The listing builds one solid part. Answer for the finished solid, in the listing's coordinates (mm). A direction names the side the tool comes from. Coordinates: 2 decimals unless noted, no trailing zeros. Loops run counter-clockwise (first coordinate to the right, second up) from the corner with the lowest first, then second, coordinate; pieces in that order, holes last. Notation, with made-up numbers: (-33, -7.5) - (-15, -7.5) arc R18 ccw to (-15, 12.5) - close; hole circle Ø7 at (29.5, 39.5). An arc over 180 degrees is marked (long way). Put each result on its own line as item: value.
```python
from build123d import *
from build123d.topology import SkipClean

# Parameters (mm, degrees)
SKETCH_1_W                       = 300
SKETCH_1_H                       = 135
SKETCH_1_R                       = 3
SM_BASE_FLANGE_1_DEPTH           = 0.7
SM_EDGE_FLANGE_1_STRIP_W         = 3.2
SM_EDGE_FLANGE_1_STRIP_H         = 0.7
SM_EDGE_FLANGE_1_STRIP_CUT_DEPTH = 300
SM_EDGE_FLANGE_1_DEPTH           = 300
SM_EDGE_FLANGE_2_STRIP_W         = 3.2
SM_EDGE_FLANGE_2_STRIP_H         = 0.7
SM_EDGE_FLANGE_2_STRIP_CUT_DEPTH = 300
SM_EDGE_FLANGE_2_DEPTH           = 300
MOVE_START                       = -0.5
MOVE_BODY_1_OUTLINE_W            = 300
MOVE_BODY_1_OUTLINE_H            = 134.3
MOVE_BODY_1_OUTLINE_R            = 3
MOVE_BODY_1_DEPTH                = 0.5
MOVE_START_2                     = -6
MOVE_BODY_1_2_OUTLINE_W          = 300
MOVE_BODY_1_2_OUTLINE_H          = 6
MOVE_BODY_1_2_DEPTH              = 4.6
MOVE_START_3                     = -1.343604
MOVE_BODY_1_3_OUTLINE_W          = 300
MOVE_BODY_1_3_OUTLINE_H          = 134.3
MOVE_BODY_1_3_OUTLINE_R          = 3
MOVE_BODY_1_3_DEPTH              = 0.643604
MOVE_BODY_1_4_OUTLINE_W          = 300
MOVE_BODY_1_4_OUTLINE_H          = 0.7
MOVE_BODY_1_4_DEPTH              = 4.2
MOVE_START_4                     = -1.4
MOVE_BODY_1_5_OUTLINE_W          = 300
MOVE_BODY_1_5_OUTLINE_H          = 134.3
MOVE_BODY_1_5_OUTLINE_R          = 3
MOVE_BODY_1_5_DEPTH              = 0.056396
MOVE_START_5                     = 3.7
MOVE_BODY_1_6_OUTLINE_W          = 300
MOVE_BODY_1_6_OUTLINE_H          = 6
MOVE_BODY_1_6_DEPTH              = 0.9
MOVE_START_6                     = -0.7
MOVE_BODY_1_7_OUTLINE_W          = 300
MOVE_BODY_1_7_OUTLINE_H          = 0.7
MOVE_BODY_1_7_DEPTH              = 0.2
MOVE_START_7                     = -151
MOVE_BODY_1_8_DEPTH              = 301


with BuildPart() as part:
    # 基体-法兰1: sheet metal written as solids
    # 草图1 → 基体-法兰1 (new body)
    with BuildSketch(Plane(origin=(0, 0, 0), x_dir=(1, 0, 0), z_dir=(0, 1, 0))):
        Rectangle(SKETCH_1_W, SKETCH_1_H)
        with Locations(Location((-144.5, -59.5, 0), (0, 0, 270))):
            Circle(SKETCH_1_R, mode=Mode.SUBTRACT)
        with Locations(Location((-144.5, -9.5, 0), (0, 0, 270))):
            Circle(SKETCH_1_R, mode=Mode.SUBTRACT)
        with Locations(Location((-144.5, 0.5, 0), (0, 0, 270))):
            Circle(SKETCH_1_R, mode=Mode.SUBTRACT)
        with Locations(Location((-144.5, 50.5, 0), (0, 0, 270))):
            Circle(SKETCH_1_R, mode=Mode.SUBTRACT)
        with Locations(Location((0, -9.5, 0), (0, 0, 270))):
            Circle(SKETCH_1_R, mode=Mode.SUBTRACT)
        with Locations(Location((0, 0.5, 0), (0, 0, 270))):
            Circle(SKETCH_1_R, mode=Mode.SUBTRACT)
        with Locations(Location((144.5, -59.5, 0), (0, 0, 90))):
            Circle(SKETCH_1_R, mode=Mode.SUBTRACT)
        with Locations(Location((144.5, -9.5, 0), (0, 0, 90))):
            Circle(SKETCH_1_R, mode=Mode.SUBTRACT)
        with Locations(Location((144.5, 0.5, 0), (0, 0, 90))):
            Circle(SKETCH_1_R, mode=Mode.SUBTRACT)
        with Locations(Location((144.5, 50.5, 0), (0, 0, 90))):
            Circle(SKETCH_1_R, mode=Mode.SUBTRACT)
    extrude(amount=-SM_BASE_FLANGE_1_DEPTH)

    # 边线-法兰1: sheet metal written as solids
    # 边线-法兰1 strip (on a plane across the edge) → 边线-法兰1 strip cut (cut)
    with BuildSketch(Plane(origin=(-150, -0.7, -67.5), x_dir=(0, 0, 1), z_dir=(1, 0, 0))):
        with Locations((-0.7, -0.35)):
            Rectangle(SM_EDGE_FLANGE_1_STRIP_W, SM_EDGE_FLANGE_1_STRIP_H)
    extrude(amount=SM_EDGE_FLANGE_1_STRIP_CUT_DEPTH, mode=Mode.SUBTRACT)

    # 边线-法兰1 section (on a plane across the edge) → 边线-法兰1 (add)
    with BuildSketch(Plane(origin=(-150, -0.7, -67.5), x_dir=(0, 0, 1), z_dir=(1, 0, 0))):
        with BuildLine():
            Line((0, 0.2), (0, 5.3))
            Line((0, 5.3), (0.7, 5.3))
            Line((0.7, 5.3), (0.7, 0.2))
            ThreePointArc((0.7, 0.2), (0.758578644, 0.058578644), (0.9, 0))
            Line((0.9, 0), (0.9, -0.7))
            ThreePointArc((0.9, -0.7), (0.263603897, -0.436396103), (0, 0.2))
        make_face()
    extrude(amount=SM_EDGE_FLANGE_1_DEPTH)

    # 边线-法兰2: sheet metal written as solids
    # 边线-法兰2 strip (on a plane across the edge) → 边线-法兰2 strip cut (cut)
    with BuildSketch(Plane(origin=(150, -6, -67.5), x_dir=(0, 1, 0), z_dir=(-1, 0, 0))):
        with Locations((-0.7, -0.35)):
            Rectangle(SM_EDGE_FLANGE_2_STRIP_W, SM_EDGE_FLANGE_2_STRIP_H)
    extrude(amount=SM_EDGE_FLANGE_2_STRIP_CUT_DEPTH, mode=Mode.SUBTRACT)

    # 边线-法兰2 section (on a plane across the edge) → 边线-法兰2 (add)
    with BuildSketch(Plane(origin=(150, -6, -67.5), x_dir=(0, 1, 0), z_dir=(-1, 0, 0))):
        with BuildLine():
            Line((0, 0.2), (0, 5.3))
            Line((0, 5.3), (0.7, 5.3))
            Line((0.7, 5.3), (0.7, 0.2))
            ThreePointArc((0.7, 0.2), (0.758578644, 0.058578644), (0.9, 0))
            Line((0.9, 0), (0.9, -0.7))
            ThreePointArc((0.9, -0.7), (0.263603897, -0.436396103), (0, 0.2))
        make_face()
    extrude(amount=SM_EDGE_FLANGE_2_DEPTH)

    # Move Body 1: read off the stored shape, not the designer's step
    # Move Body 1 outline → Move Body 1 (cut)
    with BuildSketch(Plane(origin=(0, 0, 0), x_dir=(1, 0, 0), z_dir=(0, 1, 0)).offset(MOVE_START)):
        with Locations((0, -0.35)):
            Rectangle(MOVE_BODY_1_OUTLINE_W, MOVE_BODY_1_OUTLINE_H)
        with Locations((-144.5, -59.5)):
            Circle(MOVE_BODY_1_OUTLINE_R, mode=Mode.SUBTRACT)
        with Locations((-144.5, -9.5)):
            Circle(MOVE_BODY_1_OUTLINE_R, mode=Mode.SUBTRACT)
        with Locations((-144.5, 0.5)):
            Circle(MOVE_BODY_1_OUTLINE_R, mode=Mode.SUBTRACT)
        with Locations((144.5, -59.5)):
            Circle(MOVE_BODY_1_OUTLINE_R, mode=Mode.SUBTRACT)
        with Locations((0, -9.5)):
            Circle(MOVE_BODY_1_OUTLINE_R, mode=Mode.SUBTRACT)
        with Locations((0, 0.5)):
            Circle(MOVE_BODY_1_OUTLINE_R, mode=Mode.SUBTRACT)
        with Locations((144.5, -9.5)):
            Circle(MOVE_BODY_1_OUTLINE_R, mode=Mode.SUBTRACT)
        with Locations((144.5, 0.5)):
            Circle(MOVE_BODY_1_OUTLINE_R, mode=Mode.SUBTRACT)
        with Locations((-144.5, 50.5)):
            Circle(MOVE_BODY_1_OUTLINE_R, mode=Mode.SUBTRACT)
        with Locations((144.5, 50.5)):
            Circle(MOVE_BODY_1_OUTLINE_R, mode=Mode.SUBTRACT)
    extrude(amount=MOVE_BODY_1_DEPTH, mode=Mode.SUBTRACT)

    # Move Body 1 2 outline → Move Body 1 2 (cut)
    with BuildSketch(Plane(origin=(0, 0, 0), x_dir=(1, 0, 0), z_dir=(0, 1, 0)).offset(MOVE_START_2)):
        with Locations((0, 69.8)):
            Rectangle(MOVE_BODY_1_2_OUTLINE_W, MOVE_BODY_1_2_OUTLINE_H)
    extrude(amount=MOVE_BODY_1_2_DEPTH, mode=Mode.SUBTRACT)

    # Move Body 1 3 outline → Move Body 1 3 (add)
    with SkipClean():  # the faces are left unmerged after this step: merging them gives an invalid solid
        with BuildSketch(Plane(origin=(0, 0, 0), x_dir=(1, 0, 0), z_dir=(0, 1, 0)).offset(MOVE_START_3)):
            with Locations((0, -0.35)):
                Rectangle(MOVE_BODY_1_3_OUTLINE_W, MOVE_BODY_1_3_OUTLINE_H)
            with Locations((-144.5, -59.5)):
                Circle(MOVE_BODY_1_3_OUTLINE_R, mode=Mode.SUBTRACT)
            with Locations((-144.5, -9.5)):
                Circle(MOVE_BODY_1_3_OUTLINE_R, mode=Mode.SUBTRACT)
            with Locations((-144.5, 0.5)):
                Circle(MOVE_BODY_1_3_OUTLINE_R, mode=Mode.SUBTRACT)
            with Locations((144.5, -59.5)):
                Circle(MOVE_BODY_1_3_OUTLINE_R, mode=Mode.SUBTRACT)
            with Locations((0, -9.5)):
                Circle(MOVE_BODY_1_3_OUTLINE_R, mode=Mode.SUBTRACT)
            with Locations((0, 0.5)):
                Circle(MOVE_BODY_1_3_OUTLINE_R, mode=Mode.SUBTRACT)
            with Locations((144.5, -9.5)):
                Circle(MOVE_BODY_1_3_OUTLINE_R, mode=Mode.SUBTRACT)
            with Locations((144.5, 0.5)):
                Circle(MOVE_BODY_1_3_OUTLINE_R, mode=Mode.SUBTRACT)
            with Locations((-144.5, 50.5)):
                Circle(MOVE_BODY_1_3_OUTLINE_R, mode=Mode.SUBTRACT)
            with Locations((144.5, 50.5)):
                Circle(MOVE_BODY_1_3_OUTLINE_R, mode=Mode.SUBTRACT)
        extrude(amount=MOVE_BODY_1_3_DEPTH)

    # Move Body 1 4 outline → Move Body 1 4 (add)
    with SkipClean():  # the faces are left unmerged after this step: merging them gives an invalid solid
        with BuildSketch(Plane(origin=(0, 0, 0), x_dir=(1, 0, 0), z_dir=(0, 1, 0)).offset(MOVE_START)):
            with Locations((0, 67.15)):
                Rectangle(MOVE_BODY_1_4_OUTLINE_W, MOVE_BODY_1_4_OUTLINE_H)
        extrude(amount=MOVE_BODY_1_4_DEPTH)

    # Move Body 1 5 outline → Move Body 1 5 (add)
    with SkipClean():  # the faces are left unmerged after this step: merging them gives an invalid solid
        with BuildSketch(Plane(origin=(0, 0, 0), x_dir=(1, 0, 0), z_dir=(0, 1, 0)).offset(MOVE_START_4)):
            with Locations((0, -0.35)):
                Rectangle(MOVE_BODY_1_5_OUTLINE_W, MOVE_BODY_1_5_OUTLINE_H)
            with Locations((-144.5, -59.5)):
                Circle(MOVE_BODY_1_5_OUTLINE_R, mode=Mode.SUBTRACT)
            with Locations((-144.5, -9.5)):
                Circle(MOVE_BODY_1_5_OUTLINE_R, mode=Mode.SUBTRACT)
            with Locations((-144.5, 0.5)):
                Circle(MOVE_BODY_1_5_OUTLINE_R, mode=Mode.SUBTRACT)
            with Locations((144.5, -59.5)):
                Circle(MOVE_BODY_1_5_OUTLINE_R, mode=Mode.SUBTRACT)
            with Locations((0, -9.5)):
                Circle(MOVE_BODY_1_5_OUTLINE_R, mode=Mode.SUBTRACT)
            with Locations((0, 0.5)):
                Circle(MOVE_BODY_1_5_OUTLINE_R, mode=Mode.SUBTRACT)
            with Locations((144.5, -9.5)):
                Circle(MOVE_BODY_1_5_OUTLINE_R, mode=Mode.SUBTRACT)
            with Locations((144.5, 0.5)):
                Circle(MOVE_BODY_1_5_OUTLINE_R, mode=Mode.SUBTRACT)
            with Locations((-144.5, 50.5)):
                Circle(MOVE_BODY_1_5_OUTLINE_R, mode=Mode.SUBTRACT)
            with Locations((144.5, 50.5)):
                Circle(MOVE_BODY_1_5_OUTLINE_R, mode=Mode.SUBTRACT)
        extrude(amount=MOVE_BODY_1_5_DEPTH)

    # Move Body 1 6 outline → Move Body 1 6 (add)
    with SkipClean():  # the faces are left unmerged after this step: merging them gives an invalid solid
        with BuildSketch(Plane(origin=(0, 0, 0), x_dir=(1, 0, 0), z_dir=(0, 1, 0)).offset(MOVE_START_5)):
            with Locations((0, 69.8)):
                Rectangle(MOVE_BODY_1_6_OUTLINE_W, MOVE_BODY_1_6_OUTLINE_H)
        extrude(amount=MOVE_BODY_1_6_DEPTH)

    # Move Body 1 7 outline → Move Body 1 7 (add)
    with SkipClean():  # the faces are left unmerged after this step: merging them gives an invalid solid
        with BuildSketch(Plane(origin=(0, 0, 0), x_dir=(1, 0, 0), z_dir=(0, 1, 0)).offset(MOVE_START_6)):
            with Locations((0, 67.15)):
                Rectangle(MOVE_BODY_1_7_OUTLINE_W, MOVE_BODY_1_7_OUTLINE_H)
        extrude(amount=MOVE_BODY_1_7_DEPTH)

    # Move Body 1 8 outline → Move Body 1 8 (cut)
    with BuildSketch(Plane.YZ.offset(MOVE_START_7)):
        with BuildLine():
            Line((-0.5, 67.5), (-0.7, 67.5))
            Line((-0.7, 67.5), (-0.7, -66.6))
            ThreePointArc((-0.7, -66.6), (-0.641421356, -66.741421356), (-0.5, -66.8))
            Line((-0.5, -66.8), (-0.5, 67.5))
        make_face()
        with BuildLine():
            ThreePointArc((-0.7, -67.477496439), (-1.203562364, -67.161248608), (-1.4, -66.6))
            Line((-1.4, -66.6), (-1.4, -67.5))
            Line((-1.4, -67.5), (-0.9, -67.5))
            ThreePointArc((-0.9, -67.5), (-0.799368978, -67.494356415), (-0.7, -67.477496439))
        make_face()
        with BuildLine():
            Line((4.6, -66.8), (3.7, -66.8))
            ThreePointArc((3.7, -66.8), (4.336396103, -67.063603897), (4.6, -67.7))
            Line((4.6, -67.7), (4.6, -66.8))
        make_face()
        with BuildLine():
            ThreePointArc((-0.5, -67.5), (-0.600631022, -67.494356415), (-0.7, -67.477496439))
            Line((-0.7, -67.477496439), (-0.7, -67.5))
            Line((-0.7, -67.5), (-0.5, -67.5))
        make_face()
        with BuildLine():
            ThreePointArc((3.9, -67.7), (3.841421356, -67.558578644), (3.7, -67.5))
            Line((3.7, -67.5), (3.7, -72.8))
            Line((3.7, -72.8), (3.9, -72.8))
            Line((3.9, -72.8), (3.9, -67.7))
        make_face()
    extrude(amount=MOVE_BODY_1_8_DEPTH, mode=Mode.SUBTRACT)


solid = part.part
```
1) For faces 3 (the face through (-2, -0.7, -14)), 4 (the face through (-2, 3.9, -70)), 5 (the face through (-141.64, -1.05, -1.4)), determine the directions among +Z, -Z, +X, -X, +Y, -Y from which every point of the face is accessible in a straight line to the end or side of a thin tool.
Found:
face 3: +Z, +X, -X, +Y
face 4: -Z, +X, -X, -Y
face 5: +Y, -Y
2) Each of these flat-tipped pins is pushed along its axis until it touches: pin 1 (1 mm diameter, centred on x = -74.5, y = 0.5, fed in from +Z); pin 2 (10 mm diameter, centred on x = -18.5, z = -52.5, fed in from +Y); pin 3 (5 mm diameter, centred on x = 144.5, z = -50.5, fed in from +Y); pin 4 (1.5 mm diameter, centred on x = 58, z = -71, fed in from -Y). Where does it stop, or does it pass through?
Found:
pin 1: stops at z = -66.8
pin 2: stops at y = -0.7
pin 3: passes through
pin 4: stops at y = 3.9
3) Straight lines are drawn through the part: L1, parallel to X at y = -0.9, z = -0.5; L2, parallel to X at y = -0.9, z = 59.5; L3, parallel to Z at x = -144.5, y = -0.85. For each, find the intervals that lie inside material, in ascending order. Write a range as [from, to].
Found:
L1: x = [-150, -147.5], [-141.5, -3], [3, 141.5], [147.5, 150]
L2: x = [-150, -147.5], [-141.5, 141.5], [147.5, 150]
L3: z = [-67.43, -53.5], [-47.5, -3.5], [2.5, 6.5], [12.5, 56.5], [62.5, 67.5]
4) The part is cut by section B-B (x = 0). Give the vertices of the cut face in (y, z).
Found:
outline: (-1.4, -66.6) arc R0.9 ccw to (-0.5, -67.5) - (3.7, -67.5) arc R0.2 cw to (3.9, -67.7) - (3.9, -72.8) - (4.6, -72.8) - (4.6, -67.7) arc R0.9 ccw to (3.7, -66.8) - (-0.5, -66.8) arc R0.2 cw to (-0.7, -66.6) - (-0.7, -3.5) - (-1.4, -3.5) - close; (-1.4, 2.5) - (-0.7, 2.5) - (-0.7, 6.5) - (-1.4, 6.5) - close; (-1.4, 12.5) - (-0.7, 12.5) - (-0.7, 67.5) - (-1.4, 67.5) - close
5) The part is cut by section D-D (x = 144.5). Give the vertices of the cut face in (y, z), and give its area (3 significant figures).
Found:
outline: (-1.4, -66.6) arc R0.9 ccw to (-0.5, -67.5) - (3.7, -67.5) arc R0.2 cw to (3.9, -67.7) - (3.9, -72.8) - (4.6, -72.8) - (4.6, -67.7) arc R0.9 ccw to (3.7, -66.8) - (-0.5, -66.8) arc R0.2 cw to (-0.7, -66.6) - (-0.7, -53.5) - (-1.4, -53.5) - close; (-1.4, -47.5) - (-0.7, -47.5) - (-0.7, -3.5) - (-1.4, -3.5) - close; (-1.4, 2.5) - (-0.7, 2.5) - (-0.7, 6.5) - (-1.4, 6.5) - close; (-1.4, 12.5) - (-0.7, 12.5) - (-0.7, 56.5) - (-1.4, 56.5) - close; (-1.4, 62.5) - (-0.7, 62.5) - (-0.7, 67.5) - (-1.4, 67.5) - close
area: 84.8 mm^2
6) The part is cut by section C-C (z = 59.5). Give the vertices of the cut face in (x, y).
Found:
outline: (-150, -1.4) - (-147.5, -1.4) - (-147.5, -0.7) - (-150, -0.7) - close; (-141.5, -1.4) - (141.5, -1.4) - (141.5, -0.7) - (-141.5, -0.7) - close; (147.5, -1.4) - (150, -1.4) - (150, -0.7) - (147.5, -0.7) - close
7) The part is cut by section A-A (z = -0.5). Give the vertices of the cut face in (x, y), and give its area (3 significant figures).
Found:
outline: (-150, -1.4) - (-147.5, -1.4) - (-147.5, -0.7) - (-150, -0.7) - close; (-141.5, -1.4) - (-3, -1.4) - (-3, -0.7) - (-141.5, -0.7) - close; (3, -1.4) - (141.5, -1.4) - (141.5, -0.7) - (3, -0.7) - close; (147.5, -1.4) - (150, -1.4) - (150, -0.7) - (147.5, -0.7) - close
area: 197 mm^2
8) For a pull along Z with two mould halves and no side action, classify faces 1 (the face through (150, -1, -3)), 2 (the face through (147.36, -1.05, -51.4)) as pulls with the +Z half, pulls with the -Z half, needs draft (parallel to the pull), parting line crosses it, or undercut.
Found:
face 1: needs draft
face 2: undercut
